Verification items for this drawing (mm, ordinates from the low corner). A direction names the side the tool comes from. Coordinates: 2 decimals unless noted, no trailing zeros. Write each loop counter-clockwise with the first axis right and the second up, starting at its lowest first coordinate (ties: lowest second). Pieces come first, ordered by that corner, then holes.
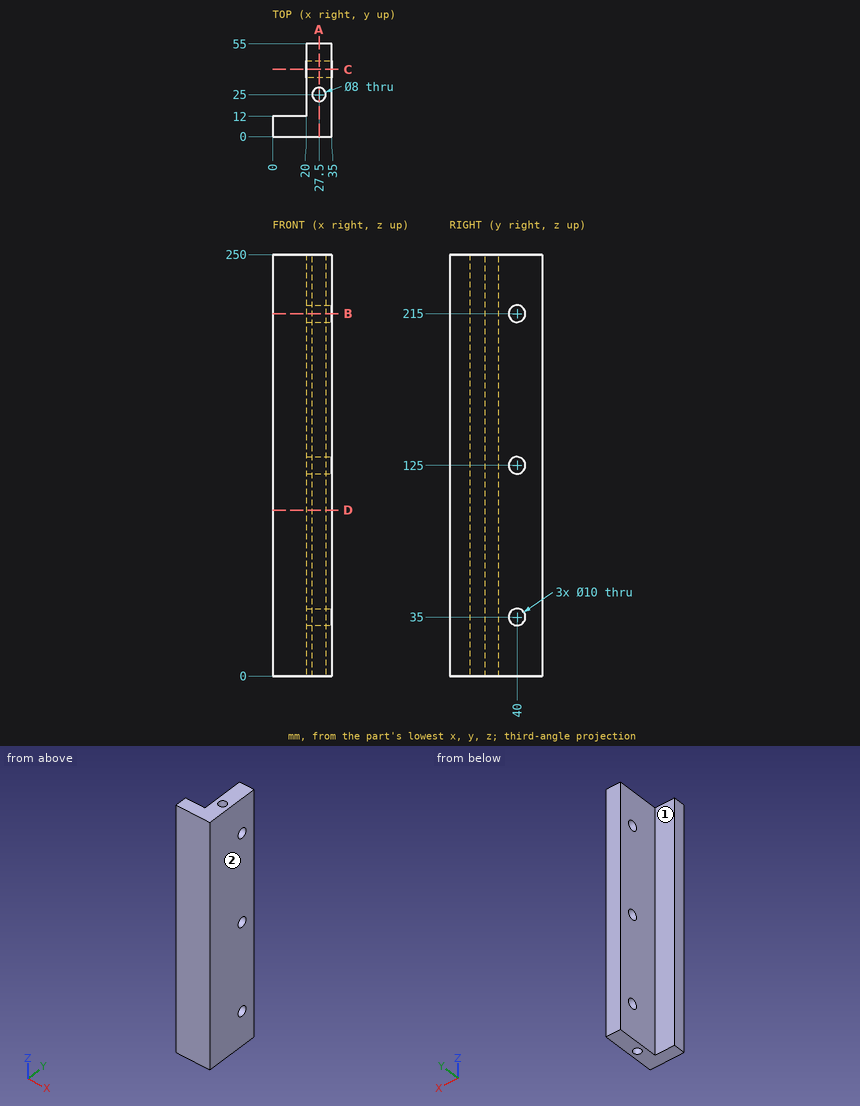
1. Thickness scan on line 1 along Z through (x, y) = (24.25, 40); line 2 along Y through (x, z) = (27.5, 144); line 3 along Y through (x, z) = (14, 172.5). Record the ranges inside material, lowest first.
Computed values:
line 1: z = 0 to 30, 40 to 120, 130 to 210, 220 to 250
line 2: y = 0 to 21, 29 to 55
line 3: y = 0 to 12
2. Access from +Z, -Z, +X, -X, +Y, -Y to the whole of each face (thin tool, end or side, straight path). Record for the marked faces 1 and 2.
Computed values:
face 1: +Z, -Z, -X, +Y
face 2: +Z, -Z, +X, +Y, -Y
3. Sectioned sample at C-C, the plane y = 40. Record the boundary of the cut face in (x, z), and give its area (3 significant figures).
Computed values:
outline: (20, 0) - (35, 0) - (35, 30) - (20, 30) - close; (20, 40) - (35, 40) - (35, 120) - (20, 120) - close; (20, 130) - (35, 130) - (35, 210) - (20, 210) - close; (20, 220) - (35, 220) - (35, 250) - (20, 250) - close
area: 3,300 mm2
4. Sectioned sample at D-D, the plane z = 98.5. Record the boundary of the cut face in (x, y), and give its area (3 significant figures).
Computed values:
outline: (0, 0) - (35, 0) - (35, 55) - (20, 55) - (20, 12) - (0, 12) - close; hole circle Ø8 at (27.5, 25)
area: 1,010 mm2
5. Sectioned sample at A-A, the plane x = 27.5. Record the boundary of the cut face in (y, z).
Computed values:
outline: (0, 0) - (21, 0) - (21, 250) - (0, 250) - close; (29, 0) - (55, 0) - (55, 250) - (29, 250) - close; hole circle Ø10 at (40, 35); hole circle Ø10 at (40, 125); hole circle Ø10 at (40, 215)
6. Gauge pin test, flat ends, axial feed: pin 1 Ø13 at (x, y) = (27.5, 25) entering from -Z; pin 2 Ø4 at (y, z) = (29, 176.5) entering from -X; pin 3 Ø1.5 at (x, z) = (17.5, 35.5) entering from +Y. Record the tip position at first contact, or that the pin passes through.
Computed values:
pin 1: stops at z = 0
pin 2: stops at x = 20
pin 3: stops at y = 12
7. Sectioned sample at B-B, the plane z = 215. Record the boundary of the cut face in (x, y).
Computed values:
outline: (0, 0) - (35, 0) - (35, 35) - (20, 35) - (20, 12) - (0, 12) - close; (20, 45) - (35, 45) - (35, 55) - (20, 55) - close; hole circle Ø8 at (27.5, 25)
